```python
from build123d import *

# Parameters (mm, degrees)
F0_W        = 23.5866680741
F0_H        = 16.0968005657
F0_W_2      = 26.164457202
F0_H_2      = 20.3793495893
F1_DEPTH    = 25.4
F2_R        = 5.08
F3_R        = 5.08
F4_T1_DEPTH = 33.02
F4_S5_W     = 5.08
F4_S5_H     = 5.08
F4_T6_DEPTH = 5.08


# Not quite as in the source:
# - a fillet or chamfer that OpenCascade refuses, or shapes differently, is made with other operations: its cross-section is extruded or revolved along the edge and cut away or added


with BuildPart() as f1:
    # F0 (on Top) → F1 (new body)
    with BuildSketch(Plane.XY):
        with Locations((-11.7933340371, -6.5704584122)):
            Rectangle(F0_W, F0_H)
        with Locations((13.082228601, 9.5263421535)):
            Rectangle(F0_W_2, F0_H)
        with Locations((-11.7933340371, 9.5263421535)):
            Rectangle(F0_W, F0_H)
        with Locations((13.082228601, 27.7644172311)):
            Rectangle(F0_W_2, F0_H_2)
        with Locations((13.082228601, -6.5704584122)):
            Rectangle(F0_W_2, F0_H)
    extrude(amount=F1_DEPTH)

    # F2
    f2_edges = [f1.edges().sort_by_distance(p)[0] for p in [
        (-23.586668, 1.477942, 0),
    ]]
    fillet(f2_edges, radius=F2_R)

    # F3
    f3_edges = [f1.edges().sort_by_distance(p)[0] for p in [
        (3.828895, -14.618859, 0),
        (-18.506668, 1.477942, 0),
        (26.164457, 11.667617, 0),
        (-9.253334, 17.574742, 0),
        (13.082229, 37.954092, 0),
        (0, 27.764417, 0),
    ]]
    fillet(f3_edges, radius=F3_R)

    # F4: fillet of radius 5.08 on 1 edges, made by hand

    # F4_s2 → F4_t1 (cut)
    with BuildSketch(Plane.XY.offset(5.08)):
        with BuildLine():
            ThreePointArc((5.08, 37.9540920258), (1.4878975516, 36.4661944742), (0, 32.8740920258))
            Line((0, 32.8740920258), (0, 37.9540920258))
            Line((0, 37.9540920258), (5.08, 37.9540920258))
        make_face()
    extrude(amount=F4_T1_DEPTH, mode=Mode.SUBTRACT)


with BuildPart() as f4_tool4:
    # F4_s5 → F4_t6 (new body)
    with BuildSketch(Plane.XZ.offset(-32.8740920258)):
        with Locations((2.54, 2.54)):
            Rectangle(F4_S5_W, F4_S5_H)
    extrude(amount=-F4_T6_DEPTH)

    # F4_s7 → F4_t8 (revolve, cut)
    with BuildSketch(Plane(origin=(5.08, 32.8740920258, 5.08), x_dir=(0.7071067812, 0, 0.7071067812), z_dir=(-0.7071067812, 0, 0.7071067812))):
        with BuildLine():
            ThreePointArc((0, -5.08), (5.08, 0), (0, 5.08))
            Line((0, 5.08), (0, -5.08))
        make_face()
    revolve(axis=Axis((5.08, 32.8740920258, 5.08), (0, 1, 0)), mode=Mode.SUBTRACT)


with BuildPart() as f1_1:
    add(f1.part)

    # F4_t3: cut F4_tool4
    add(f4_tool4.part, mode=Mode.SUBTRACT)


solid = f1_1.part
```
The listing builds one solid part. Answer for the finished solid, in the listing's coordinates (mm). A direction names the side the tool comes from. Coordinates: 2 decimals unless noted, no trailing zeros. Order: outer loops, then holes, each group sorted by start corner. A loop starts at its lowest first (then second) coordinate and runs counter-clockwise, first axis right, second up. Notation, with made-up numbers: M 63.25,88.5 L 116.25,88.5 A18 ccw 116.25,123.5 Z; hole C -11.75,19.5 d7. An arc over 180 degrees is marked long. Answer as a JSON object with one key per item and string values. Group by question number.
1. Section B-B on z = 13.25 is taken. Write down the section's boundary in (x, y), then the cut area to 3 significant figures.
2. Section A-A on y = 28.5 is taken. Write down the section's boundary in (x, z).
3. Section D-D on z = 1.75 is taken. Write down the section's boundary in (x, y).
4. Straight lines are drawn through the part: line 1 (Y direction, x = -3, z = 24.75); line 2 (X direction, y = 18, z = 20.5); line 3 (X direction, y = 9.5, z = 1). For each, find the intervals that lie inside material, in ascending order.
5. A tool of negligible diameter and unlimited length cuts with its end or side. For faces 1 (the cylindrical face through (-9.5, 16.05, 1.45)), 2 (the flat face through (6, 6, 25.4)), 3 (the flat face through (0, 25, 15)), from which of +Z, -Z, +X, -X, +Y, -Y can it reach the whole face along a straight path? Write none if from no direction.
6. Section C-C on x = -8 is taken. Write down the section's boundary in (y, z).
7. Flat-ended cylindrical pins translate along their axes: P1, Ø5.5, axis at x = -5.5, z = 18.5, coming from the +Y side; P2, Ø2, axis at y = 23.5, z = 3.5, coming from the -X side; P3, Ø5, axis at x = -2, z = 17.5, coming from the +Y side. Find the tip coordinate at first contact, or state that the pin passes through.
Values follow:
{
 "1": {"outline": "M -23.59,-9.54 A5.08 ccw -18.51,-14.62 L 26.16,-14.62 L 26.16,37.95 L 5.08,37.95 A5.08 ccw 0,32.87 L 0,17.57 L -18.51,17.57 A5.08 ccw -23.59,12.49 Z", "area": "2,120 mm2"},
 "2": {"outline": "M 0,5.08 A5.08 ccw 5.08,0 L 21.08,0 A5.08 ccw 26.16,5.08 L 26.16,25.4 L 0,25.4 Z"},
 "3": {"outline": "M -22.34,-9.54 A3.84 ccw -18.51,-13.38 L 24.92,-13.38 L 24.92,36.71 L 5.08,36.71 A3.84 ccw 1.24,32.87 L 1.24,16.33 L -18.51,16.33 A3.84 ccw -22.34,12.49 Z"},
 "4": {"line 1": "-14.62 to 17.57", "line 2": "0 to 26.16", "line 3": "-21.53 to 24.11"},
 "5": {"face 1": "-Z, -X, +Y", "face 2": "+Z, +X, -X, +Y, -Y", "face 3": "+Z, -Z, -X, +Y"},
 "6": {"outline": "M -14.62,5.08 A5.08 ccw -9.54,0 L 12.49,0 A5.08 ccw 17.57,5.08 L 17.57,25.4 L -14.62,25.4 Z"},
 "7": {"P1": "y = 17.57", "P2": "x = 0.03", "P3": "y = 35.07"}
}
